from build123d import *

# Parameters (mm, degrees)
F_3_8_CLEARANCE_HOLE1_D     = 10.0838
F_3_8_CLEARANCE_HOLE1_DEPTH = 25.4
SKETCH6_R                   = 11.1125
CUT_EXTRUDE1_DEPTH          = 7.112
SKETCH7_R                   = 11.1125
CUT_EXTRUDE2_DEPTH          = 12.065


with BuildPart() as part:
    # Sketch1 → Revolve1 (revolve)
    with BuildSketch(Plane(origin=(0, 0, 0), x_dir=(0, 0, -1), z_dir=(1, 0, 0))):
        Polygon((0, 0), (0, 14.2875), (9.652, 14.2875), (9.652, 19.05), (15.748, 19.05), (15.748, 14.2875), (25.4, 14.2875), (25.4, 0), align=None)
    revolve(axis=Axis((0, 0, 13.696708861), (0, 0, -1)))

    # 3/8 Clearance Hole1
    with Locations(Plane.XY):
        with Locations((0, 0)):
            Hole(F_3_8_CLEARANCE_HOLE1_D / 2, depth=F_3_8_CLEARANCE_HOLE1_DEPTH)

    # Sketch6 → Cut-Extrude1 (cut)
    with BuildSketch(Plane.XY):
        Circle(SKETCH6_R)
    extrude(amount=-CUT_EXTRUDE1_DEPTH, mode=Mode.SUBTRACT)

    # Sketch7 → Cut-Extrude2 (cut)
    with BuildSketch(Plane(origin=(0, 0, -25.4), x_dir=(-1, 0, 0), z_dir=(0, 0, -1))):
        Circle(SKETCH7_R)
    extrude(amount=-CUT_EXTRUDE2_DEPTH, mode=Mode.SUBTRACT)


solid = part.part
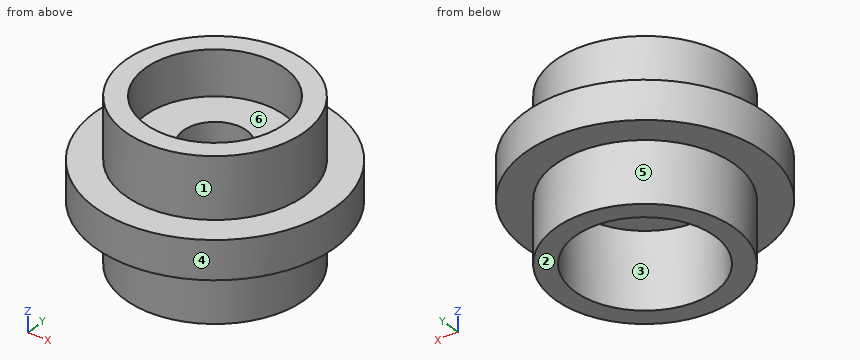
The listing builds one solid part. Answer for the finished solid, in the listing's coordinates (mm). Face numbers are marked on the shaded views. A direction names the side the tool comes from. Round coordinates to 2 decimals unless told otherwise and drop trailing zeros. Write each loop counter-clockwise with the first axis right and the second up, starting at its lowest first coordinate (ties: lowest second). Pieces come first, ordered by that corner, then holes. Notation, with made-up numbers: (55, 51.5) - (74, 51.5) arc R20 cw to (74, 65.5) - close; hole circle Ø4 at (62.25, 21.5). An arc over 180 degrees is marked (long way). Use a Markdown table: item, result. Add a question column.
1. A tool of negligible diameter and unlimited length cuts with its end or side. For the marked faces 4, 5 and 6, from which of +Z, -Z, +X, -X, +Y, -Y can it reach the whole face along a straight path? Write none if from no direction.
2. Consider line 1 (Z direction, x = -1.5, y = -10) (3 decimals); line 2 (Y direction, x = 8, z = -15.25); line 3 (Z direction, x = -14.5, y = 3). Determine where each line is inside the solid, lowest interval first.
3. For a pull along X with two mould halves and no side action, classify the marked faces 1, 2 and 3 as +X half, -X half, draft (parallel to the pull), parting line (faces both ways), or undercut.
4. Flat-ended cylindrical pins translate along their axes: P1, Ø2, axis at x = 4, z = -16.5, coming from the -Y side; P2, Ø18, axis at x = 0, y = 0, coming from the -Z side (3 decimals); P3, Ø8, axis at x = -5.5, y = 1.5, coming from the +Z side. Find the tip coordinate at first contact, or state that the pin passes through.
5. The part is cut by section C-C (y = 12). Write down the section's boundary in (x, z).
Reported:
| question | item | result |
|---|---|---|
| 1 | face 4 | +Z, -Z |
| 1 | face 5 | -Z |
| 1 | face 6 | +Z |
| 2 | line 1 | -13.335 to -7.112 |
| 2 | line 2 | -17.29 to -7.71, 7.71 to 17.29 |
| 2 | line 3 | -15.75 to -9.65 |
| 3 | face 1 | parting line |
| 3 | face 2 | draft |
| 3 | face 3 | undercut |
| 4 | P1 | y = -18.75 |
| 4 | P2 | z = -13.335 |
| 4 | P3 | z = -7.11 |
| 5 | outline | (-14.8, -15.75) - (-7.75, -15.75) - (-7.75, -25.4) - (7.75, -25.4) - (7.75, -15.75) - (14.8, -15.75) - (14.8, -9.65) - (7.75, -9.65) - (7.75, 0) - (-7.75, 0) - (-7.75, -9.65) - (-14.8, -9.65) - close |
